CAD build for the part. Positions are in the model's coordinates, mm. A direction names the side the tool comes from. Give positions to 0.01 mm unless a question says otherwise; leave off trailing zeros. Order: outer loops, then holes, each group sorted by start corner. A loop starts at its lowest first (then second) coordinate and runs counter-clockwise, first axis right, second up. Notation, with made-up numbers: M 1,-36.5 L 37,-36.5 A22 cw 37,-19.5 Z; hole C 71.25,36 d2. An arc over 180 degrees is marked long. Put each result on its own line as item: value. Start each with the question number.
1) Tool access for faces 1 (the face through (4.3, -2.1, 0)), 2 (the face through (-2.17, -9.76, 0.99)): list every direction of +Z, -Z, +X, -X, +Y, -Y with a clear straight run to the whole face (end or side of a thin tool).
2) Cut at D-D (y = -8). Write the cut outline in (x, z), and give its area (3 significant figures).
3) Two-plate mould, pull along X, no slides. Class faces 3 (the face through (0.867, -3.905, -0.788)), 4 (the face through (0.59, 4.46, -1.73)), 5 (the face through (3, -3, -3.5)): released by +X, released by -X, zero draft, split by the parting line, or undercut.
4) Cut at A-A (x = 0). Write the cut outline in (y, z).
5) Drill centre lines: line 1 (Y direction, x = 0, z = -1.25); line 2 (Y direction, x = 0, z = 0.5); line 3 (Z direction, x = 4, y = -8.5). Where is each one in solid material? Low to high. Write a range as [from, to].
6) Cut at C-C (z = -0.85). Write the cut outline in (x, y).
7) Pin check, flat tips, straight feed: pin 1 (1.5 mm diameter, centred on x = -4.5, z = -2.5, fed in from -Y); pin 2 (7 mm diameter, centred on x = 0, y = 0, fed in from -Z). Stop position of each tip, or through.
```python
from build123d import *

# Parameters (mm, degrees)
SKETCH1_R           = 10
BOSS_EXTRUDE1_DEPTH = 2
SKETCH2_R           = 4.5
BOSS_EXTRUDE2_DEPTH = 3.5
SKETCH3_R           = 4
CUT_EXTRUDE1_DEPTH  = 6.5


with BuildPart() as part:
    # Sketch1 → Boss-Extrude1 (new body)
    with BuildSketch(Plane.XY):
        Circle(SKETCH1_R)
    extrude(amount=BOSS_EXTRUDE1_DEPTH)

    # Sketch2 → Boss-Extrude2 (add)
    with BuildSketch(Plane(origin=(0, 0, 0), x_dir=(-1, 0, 0), z_dir=(0, 0, -1))):
        Circle(SKETCH2_R)
    extrude(amount=BOSS_EXTRUDE2_DEPTH)

    # Sketch3 → Cut-Extrude1 (cut, through all)
    with BuildSketch(Plane(origin=(0, 0, -3.5), x_dir=(-1, 0, 0), z_dir=(0, 0, -1))):
        Circle(SKETCH3_R)
    extrude(amount=-CUT_EXTRUDE1_DEPTH, mode=Mode.SUBTRACT)


solid = part.part
```
Solution:
1. face 1: -Z
1. face 2: +Z, -Z
2. outline: M -6,0 L 6,0 L 6,2 L -6,2 Z
2. area: 24.0 mm²
3. face 3: undercut
3. face 4: split by the parting line
3. face 5: zero draft
4. outline: M -10,0 L -4.5,0 L -4.5,-3.5 L -4,-3.5 L -4,2 L -10,2 Z; M 4,-3.5 L 4.5,-3.5 L 4.5,0 L 10,0 L 10,2 L 4,2 Z
5. line 1: [-4.5, -4], [4, 4.5]
5. line 2: [-10, -4], [4, 10]
5. line 3: [0, 2]
6. outline: C 0,0 d9; hole C 0,0 d8
7. pin 1: y = -2.49
7. pin 2: through
